Input: part model. Units: mm. Frame: model coordinates. Face numbers are marked on the shaded views. A direction names the side the tool comes from. Round coordinates to 2 decimals unless told otherwise and drop trailing zeros. Write each loop counter-clockwise with the first axis right and the second up, starting at its lowest first coordinate (ties: lowest second). Pieces come first, ordered by that corner, then holes. Notation, with made-up numbers: (88.5, 0) - (143.5, 0) arc R27 ccw to (143.5, 19) - close; hole circle Ø5 at (57.25, -8.5). An arc over 180 degrees is marked (long way). Use one line per item in the form item = value.
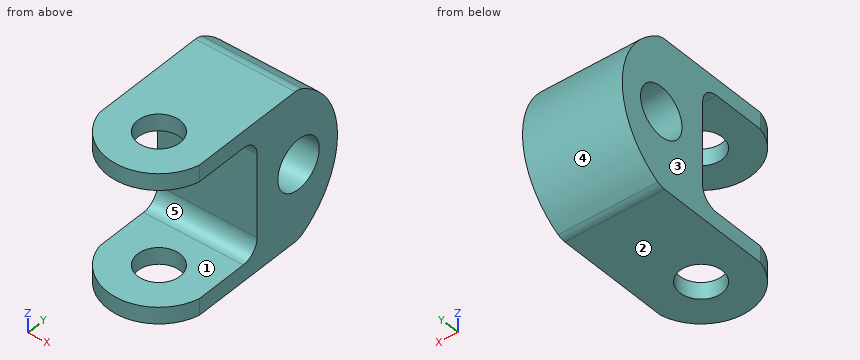
```python
from build123d import *

# Parameters (mm, degrees)
ESQUISSE1_R             = 15
BOSS_EXTRU_1_DEPTH      = 60
ESQUISSE2_R             = 12.75
ENL_V_MAT_EXTRU_1_DEPTH = 148.309198627
CONG_1_R                = 10


with BuildPart() as part:
    # Esquisse1 → Boss.-Extru.1 (new body)
    with BuildSketch(Plane(origin=(0, 0, 0), x_dir=(0, 0, -1), z_dir=(1, 0, 0))):
        with BuildLine():
            ThreePointArc((-45, 0), (0, 28.205505282), (45, 0))
            Line((45, 0), (45, -100))
            Line((45, -100), (35, -100))
            Line((35, -100), (35, -30))
            Line((35, -30), (-35, -30))
            Line((-35, -30), (-35, -100))
            Line((-35, -100), (-45, -100))
            Line((-45, -100), (-45, 0))
        make_face()
        with Locations(Location((0, 0, 0), (0, 0, 180))):
            Circle(ESQUISSE1_R, mode=Mode.SUBTRACT)
    extrude(amount=BOSS_EXTRU_1_DEPTH)

    # Esquisse2 → Enl_v. mat.-Extru.1 (cut, through all)
    with BuildSketch(Plane(origin=(0, 0, -45), x_dir=(-1, 0, 0), z_dir=(0, 0, -1))):
        with Locations(Location((-30, -65, 0), (0, 0, 90))):
            Circle(ESQUISSE2_R)
        with BuildLine():
            Line((-60, -71.861434349), (-96.965788421, -71.861434349))
            Line((-96.965788421, -71.861434349), (-96.965788421, -138.438192961))
            Line((-96.965788421, -138.438192961), (33.77611945, -138.438192961))
            Line((33.77611945, -138.438192961), (33.77611945, -71.861434349))
            Line((33.77611945, -71.861434349), (0, -71.861434349))
            ThreePointArc((0, -71.861434349), (-30, -95.774653228), (-60, -71.861434349))
        make_face()
    extrude(amount=-ENL_V_MAT_EXTRU_1_DEPTH, mode=Mode.SUBTRACT)

    # Cong_1
    cong_1_edges = [part.edges().sort_by_distance(p)[0] for p in [
        (30, 0, -45),
        (30, -30, -35),
        (30, -30, 35),
        (30, 0, 45),
    ]]
    fillet(cong_1_edges, radius=CONG_1_R)


solid = part.part
```
(1) First-contact query: pin 1 Ø15.5 at (x, y) = (30, -65) entering from +Z; pin 2 Ø12 at (x, z) = (36.5, 0) entering from -Y; pin 3 Ø12 at (x, z) = (8, -34) entering from -Y. Flat tips, straight axial feed; report the tip coordinate or a pass-through.
Derived:
pin_1 = through
pin_2 = -30
pin_3 = -91.24
(2) Cut plane C-C on z = 0. Output: boundary loops of the cut face in (x, y), then the cut area to 3 significant figures.
Derived:
outline = (0, -30) - (60, -30) - (60, -15) - (0, -15) - close; (0, 15) - (60, 15) - (60, 28.21) - (0, 28.21) - close
area = 1,690 mm^2
(3) Cut plane B-B on y = -65. Output: boundary loops of the cut face in (x, z).
Derived:
outline = (0, -45) - (17.25, -45) - (17.25, -35) - (0, -35) - close; (0, 35) - (17.25, 35) - (17.25, 45) - (0, 45) - close; (42.75, -45) - (60, -45) - (60, -35) - (42.75, -35) - close; (42.75, 35) - (60, 35) - (60, 45) - (42.75, 45) - close
(4) Draft query along Z for the marked faces 3, 4 and 5. Return one class per face: released by +Z, released by -Z, zero draft, split by the parting line, or undercut.
Derived:
face_3 = zero draft
face_4 = split by the parting line
face_5 = undercut
(5) Cut plane D-D on y = -5.5. Output: boundary loops of the cut face in (x, z), then the cut area to 3 significant figures.
Derived:
outline = (0, -45) - (60, -45) - (60, -13.96) - (0, -13.96) - close; (0, 13.96) - (60, 13.96) - (60, 45) - (0, 45) - close
area = 3,730 mm^2
(6) Access query for the marked faces 1 and 2. Directions: +Z, -Z, +X, -X, +Y, -Y. A direction counts if a zero-diameter tool reaches every point of the face in a straight line with its end or side. Return the directions, or none.
Derived:
face_1 = +X, -X, -Y
face_2 = -Z, +X, -X, +Y, -Y
(7) Cut plane A-A on x = 30. Output: boundary loops of the cut face in (y, z).
Derived:
outline = (-95.77, -45) - (-77.75, -45) - (-77.75, -35) - (-95.77, -35) - close; (-95.77, 35) - (-77.75, 35) - (-77.75, 45) - (-95.77, 45) - close; (-52.25, -45) - (-2.43, -45) arc R10 ccw to (2.41, -43.75) arc R50 ccw to (2.41, 43.75) arc R10 ccw to (-2.43, 45) - (-52.25, 45) - (-52.25, 35) - (-40, 35) arc R10 cw to (-30, 25) - (-30, -25) arc R10 cw to (-40, -35) - (-52.25, -35) - close; hole circle Ø30 at (0, 0)
(8) Material intervals for L1, parallel to Z at x = 14.5, y = -41.5; L2, parallel to X at y = -65, z = 37; L3, parallel to Y at x = 38.5, z = 0, sorted ascending.
Derived:
L1 = -45 to -35, 35 to 45
L2 = 0 to 17.25, 42.75 to 60
L3 = -30 to -15, 15 to 28.21
